Geometry check sheet. Reference: the model listing, model coordinates, mm. A direction names the side the tool comes from. Give positions to 0.01 mm unless a question says otherwise; leave off trailing zeros. Order: outer loops, then holes, each group sorted by start corner. A loop starts at its lowest first (then second) coordinate and runs counter-clockwise, first axis right, second up. Notation, with made-up numbers: M 16.5,-3 L 28.5,-3 A15 ccw 28.5,13 Z; hole C 81,28 d10. An arc over 180 degrees is marked long. Put each result on its own line as item: value. Start each with the question number.
Q1. Section check A-A on z = -3.75. Record the cut outline in (x, y).
Q2. Go/stop test with flat-tipped pins: pin 1 (1.6 mm diameter, centred on x = 21, z = -28, fed in from -Y); pin 2 (2.5 mm diameter, centred on x = 20.5, y = -3.99, fed in from +Z); pin 3 (0.8 mm diameter, centred on y = -8.5, z = -24.5, fed in from -X); pin 4 (1 mm diameter, centred on x = 21.5, z = -3, fed in from -Y). Record where each tip stops, or that it passes through.
Q3. Section check C-C on y = -17.75. Record the cut outline in (x, z), then the cut area to 3 significant figures.
Q4. Section check B-B on y = -3. State how many separate pieces and enclosed holes the cut face has, then the cut area to 3 significant figures.
Q5. Mould release check, pull along Y, two halves, no side actions. Record for faces 1 (the cylindrical face through (26.74, -8.758, -14.79)), 2 (the flat face through (24, -9, 0)), 3 (the cylindrical face through (24.31, -12.4, -14.79)), 4 (the flat face through (22, -9.189, -4)): +Y half, -Y half, draft (parallel to the pull), parting line (faces both ways), or undercut.
Q6. Access from +Z, -Z, +X, -X, +Y, -Y to the whole of each face (thin tool, end or side, straight path). Record for faces 5 (the conical face through (18.866, -3.917, -23.458)), 6 (the conical face through (19.29, -2.88, -28.57)), 7 (the flat face through (22, -9.189, -26)).
Q7. Material ranges on L1, parallel to Z at x = 21.75, y = -1; L2, parallel to Y at x = 20.25, z = -3.25; L3, parallel to Y at x = 25.5, z = -10.5, recorded low to high.
```python
from build123d import *
from OCP.BRepFilletAPI import BRepFilletAPI_MakeChamfer

# Parameters (mm, degrees)
SKETCH1_R           = 3
SKETCH1_R_2         = 1.5
BOSS_EXTRUDE1_DEPTH = 30
SKETCH1_5_R         = 4.5
SKETCH1_5_R_2       = 1.5
SKETCH1_5_W         = 2.035294118
SKETCH1_5_H         = 0.7
BOSS_EXTRUDE2_DEPTH = 8
LPATTERN1_COUNT     = 2
LPATTERN1_PITCH     = 22
CHAMFER1_SIZE       = 0.5
CHAMFER1_SIZE2      = 2
CHAMFER2_SIZE       = 2
CHAMFER2_SIZE2      = 0.5
CHAMFER3_SIZE       = 2
CHAMFER3_SIZE2      = 0.5


with BuildPart() as part:
    # Sketch1 → Boss-Extrude1 (new body)
    # profile 1 of 3: a face of its own
    with BuildSketch(Plane.XY):
        Polygon((22, -14.489354466), (25.413127335, -16.575154503), (19.913127335, -25.575154503), (16.5, -23.489354466), align=None)
    # profile 2 of 3: a face of its own
    with BuildSketch(Plane.XY):
        with BuildLine():
            Line((22.535294118, -11.030530936), (22, -14.489354466))
            Line((22, -14.489354466), (25.413127335, -16.575154503))
            Line((25.413127335, -16.575154503), (27.892093962, -13.2998479))
            ThreePointArc((27.892093962, -13.2998479), (24.329777383, -14.251704738), (22.535294118, -11.030530936))
        make_face()
    # profile 3 of 3: a face of its own
    with BuildSketch(Plane.XY):
        with Locations((25.5, -11.489354466)):
            Circle(SKETCH1_R)
        with Locations((25.5, -11.489354466)):
            Circle(SKETCH1_R_2, mode=Mode.SUBTRACT)
    extrude(amount=-BOSS_EXTRUDE1_DEPTH)

    # Sketch1<5> → Boss-Extrude2 (add)
    # profile 1 of 3: a face of its own
    with BuildSketch(Plane.XY):
        with BuildLine():
            Line((22.535294118, -9.189354466), (22.535294118, -11.030530936))
            ThreePointArc((22.535294118, -11.030530936), (25.730089497, -8.498191009), (28.5, -11.489354466))
            ThreePointArc((28.5, -11.489354466), (28.497587401, -11.609644848), (28.490353483, -11.729741755))
            Line((28.490353483, -11.729741755), (29.076489945, -4.438361169))
            Line((29.076489945, -4.438361169), (23.055037361, -0.285061809))
            ThreePointArc((23.055037361, -0.285061809), (24.484198045, -1.897425705), (25, -3.989354466))
            ThreePointArc((25, -3.989354466), (23.681980515, -7.171334981), (20.5, -8.489354466))
            Line((20.5, -8.489354466), (22.535294118, -8.489354466))
            Line((22.535294118, -8.489354466), (22.535294118, -9.189354466))
        make_face()
    # profile 2 of 3: a face of its own
    with BuildSketch(Plane.XY):
        with Locations((20.5, -3.989354466)):
            Circle(SKETCH1_5_R)
        with Locations((20.5, -3.989354466)):
            Circle(SKETCH1_5_R_2, mode=Mode.SUBTRACT)
    # profile 3 of 3: a face of its own
    with BuildSketch(Plane.XY):
        with Locations((21.517647059, -8.839354466)):
            Rectangle(SKETCH1_5_W, SKETCH1_5_H)
    boss_extrude2 = extrude(amount=-BOSS_EXTRUDE2_DEPTH)

    # LPattern1: Boss-Extrude2 ×2
    with Locations(*[(0, 0, -i * LPATTERN1_PITCH) for i in range(1, LPATTERN1_COUNT)]):
        add(boss_extrude2)

    # Chamfer1: one chamfer whose edges measure the first distance from different faces: ONE call of the kernel's chamfer builder (chamfer() names one face for all edges)
    chamfer1_edges_1 = [part.edges().sort_by_distance(p)[0] for p in [
        (19, -3.989354466, 0),
    ]]
    chamfer1_side_1 = [part.faces().sort_by_distance(p)[0] for p in [
        (22.584533606, -10.229298643, 0),
    ]]
    chamfer1_edges_2 = [part.edges().sort_by_distance(p)[0] for p in [
        (19, -3.989354466, -22),
    ]]
    chamfer1_side_2 = [part.faces().sort_by_distance(p)[0] for p in [
        (22.505894665, -4.865120782, -22),
    ]]
    chamfer1 = BRepFilletAPI_MakeChamfer(part.part.solid().wrapped)
    for e in chamfer1_edges_1:
        chamfer1.Add(CHAMFER1_SIZE, CHAMFER1_SIZE2, e.wrapped, chamfer1_side_1[0].wrapped)  # the first distance lies on this face
    for e in chamfer1_edges_2:
        chamfer1.Add(CHAMFER1_SIZE, CHAMFER1_SIZE2, e.wrapped, chamfer1_side_2[0].wrapped)  # the first distance lies on this face
    add(Compound.cast(chamfer1.Shape()), mode=Mode.REPLACE)

    # Chamfer2
    chamfer2_edges = [part.edges().sort_by_distance(p)[0] for p in [
        (19, -3.989354466, -8),
    ]]
    chamfer2_side = [part.faces().sort_by_distance(p)[0] for p in [
        (19, -3.989354466, -5),
    ]]
    chamfer(chamfer2_edges, length=CHAMFER2_SIZE, length2=CHAMFER2_SIZE2, reference=chamfer2_side[0])

    # Chamfer3
    chamfer3_edges = [part.edges().sort_by_distance(p)[0] for p in [
        (19, -3.989354466, -30),
    ]]
    chamfer3_side = [part.faces().sort_by_distance(p)[0] for p in [
        (19, -3.989354466, -27),
    ]]
    chamfer(chamfer3_edges, length=CHAMFER3_SIZE, length2=CHAMFER3_SIZE2, reference=chamfer3_side[0])


solid = part.part
```
Results found:
1. outline: M 16.5,-23.49 L 19.91,-25.58 L 25.41,-16.58 L 27.89,-13.3 A3 ccw 28.49,-11.73 L 29.08,-4.44 L 23.06,-0.29 A4.5 ccw long 20.5,-8.49 L 20.5,-9.19 L 22.54,-9.19 L 22.54,-11.03 L 22,-14.49 Z; hole C 20.5,-3.99 d3; hole C 25.5,-11.49 d3
2. pin 1: stops at y = -25.11
2. pin 2: passes through
2. pin 3: stops at x = 18.67
2. pin 4: stops at y = -23.8
3. outline: M 20.01,-30 L 24.7,-30 L 24.7,0 L 20.01,0 Z
3. area: 141 mm^2
4. separate pieces: 4
4. enclosed holes: 0
4. area: 133 mm^2
5. face 1: parting line
5. face 2: draft
5. face 3: undercut
5. face 4: undercut
6. face 5: none
6. face 6: -Z
6. face 7: +Z, -Z, -X
7. L1: z = -30 to -22, -8 to 0
7. L2: y = -25.02 to -17.35, -8.48 to -5.47, -2.51 to 0.5
7. L3: y = -16.46 to -12.99, -9.99 to -8.49
